```python
from build123d import *

# Parameters (mm, degrees)
EXTRUDE1_DEPTH             = 250
EXTRUDE2_REACH             = 252.125
SKETCH2_R                  = 1.75
SKETCH_R                   = 3
SKETCH_R_2                 = 1.75
EXTRUDE4_DEPTH             = 3.5
CHAMFER1_SIZE              = 0.2
LPATTERN1_COUNT            = 13
LPATTERN1_PITCH            = 20
CHAMFER1_OF_LPATTERN1_SIZE = 0.2


with BuildPart() as part:
    # Sketch1 → Extrude1 (new body)
    with BuildSketch(Plane.XY):
        with BuildLine():
            Line((-4.3, -3.25), (4.3, -3.25))
            Line((4.3, -3.25), (4.5, -3.05))
            Line((4.5, -3.05), (4.5, 0.455012563))
            ThreePointArc((4.5, 0.455012563), (3.924845827, 0.712323349), (3.617735397, 1.2625))
            Line((3.617735397, 1.2625), (3.15008224, 1.2625))
            Line((3.15008224, 1.2625), (3.15008224, 1.7625))
            Line((3.15008224, 1.7625), (3.65008224, 1.7625))
            ThreePointArc((3.65008224, 1.7625), (3.973877727, 2.229724887), (4.5, 2.444987437))
            Line((4.5, 2.444987437), (4.5, 3.05))
            Line((4.5, 3.05), (4.3, 3.25))
            Line((4.3, 3.25), (-4.3, 3.25))
            Line((-4.3, 3.25), (-4.5, 3.05))
            Line((-4.5, 3.05), (-4.5, 2.444987437))
            ThreePointArc((-4.5, 2.444987437), (-3.973877727, 2.229724887), (-3.65008224, 1.7625))
            Line((-3.65008224, 1.7625), (-3.15008224, 1.7625))
            Line((-3.15008224, 1.7625), (-3.15008224, 1.2625))
            Line((-3.15008224, 1.2625), (-3.617735397, 1.2625))
            ThreePointArc((-3.617735397, 1.2625), (-3.924845827, 0.712323349), (-4.5, 0.455012563))
            Line((-4.5, 0.455012563), (-4.5, -3.05))
            Line((-4.5, -3.05), (-4.3, -3.25))
        make_face()
    extrude(amount=EXTRUDE1_DEPTH)

    # Sketch2 → Extrude2 (cut, up to next)
    with BuildSketch(Plane(origin=(0, 3.25, 0), x_dir=(1, 0, 0), z_dir=(0, 1, 0)), mode=Mode.PRIVATE) as extrude2_sk1:
        with Locations(Location((0, -5, 0), (0, 0, 270))):
            Circle(SKETCH2_R)
    extrude2_tool1 = extrude(extrude2_sk1.sketch, amount=-EXTRUDE2_REACH, mode=Mode.PRIVATE) & part.part
    extrude2 = extrude2_tool1.solids().sort_by_distance((0, 3.25, 5))[0]
    add(extrude2, mode=Mode.SUBTRACT)

    # Sketch → Extrude4 (cut)
    with BuildSketch(Plane(origin=(0, 3.25, 0), x_dir=(1, 0, 0), z_dir=(0, 1, 0))):
        with Locations(Location((0, -5, 0), (0, 0, 270))):
            Circle(SKETCH_R)
        with Locations(Location((0, -5, 0), (0, 0, 270))):
            Circle(SKETCH_R_2, mode=Mode.SUBTRACT)
    extrude4 = extrude(amount=-EXTRUDE4_DEPTH, mode=Mode.SUBTRACT)

    # Chamfer1
    chamfer1_edges = [part.edges().sort_by_distance(p)[0] for p in [
        (0, -3.25, 3.25),
        (0, 3.25, 2),
    ]]
    chamfer(chamfer1_edges, length=CHAMFER1_SIZE)

    # LPattern1: Extrude2, Extrude4 ×13
    with Locations(*[(0, 0, i * LPATTERN1_PITCH) for i in range(1, LPATTERN1_COUNT)]):
        add(extrude2, mode=Mode.SUBTRACT)
        add(extrude4, mode=Mode.SUBTRACT)

    # Chamfer1 of LPattern1
    chamfer1_of_lpattern1_edges = [part.edges().sort_by_distance(p)[0] for p in [
        (0, -3.25, 23.25),
        (0, 3.25, 22),
        (0, -3.25, 43.25),
        (0, 3.25, 42),
        (0, -3.25, 63.25),
        (0, 3.25, 62),
        (0, -3.25, 83.25),
        (0, 3.25, 82),
        (0, -3.25, 103.25),
        (0, 3.25, 102),
        (0, -3.25, 123.25),
        (0, 3.25, 122),
        (0, -3.25, 143.25),
        (0, 3.25, 142),
        (0, -3.25, 163.25),
        (0, 3.25, 162),
        (0, -3.25, 183.25),
        (0, 3.25, 182),
        (0, -3.25, 203.25),
        (0, 3.25, 202),
        (0, -3.25, 223.25),
        (0, 3.25, 222),
        (0, -3.25, 243.25),
        (0, 3.25, 242),
    ]]
    chamfer(chamfer1_of_lpattern1_edges, length=CHAMFER1_OF_LPATTERN1_SIZE)


solid = part.part
```
Here's how the part is built. I have some questions about the finished solid (model axes, mm). Coordinates: 2 decimals unless noted, no trailing zeros. Answer as a JSON object with one key per item and string values. Group by question number.
(1) I need wall thicknesses on probe 1 along Y at (x, z) = (3.25, 54.5); probe 2 along X at (y, z) = (-1.7, 25); probe 3 along X at (y, z) = (1.35, 65). Which ranges of each line are inside material? Lowest first, please.
(2) Suppose I cut it at A-A, the plane x = 0. State how many separate pieces and enclosed holes the cut face has, then the cut area to 3 significant figures.
(3) For pin 1 (4 mm diameter, centred on x = 0, z = 105, fed in from +Y); pin 2 (3 mm diameter, centred on x = 0, z = 65, fed in from +Y), each with a flat end and sliding along its axis, tell me the tip position at first contact or that it passes through.
(4) If we mould it in two halves opening along Z, with no side actions, what happens to faces 1 (the face through (0, 1, 242)), 2 (the face through (0, 0, 0))? For each: released by +Z, released by -Z, zero draft, split by the parting line, or undercut.
Values found:
{
 "1": {"probe 1": "y = -3.25 to 1.26, 1.76 to 3.25", "probe 2": "x = -4.5 to -1.75, 1.75 to 4.5", "probe 3": "x = -3.15 to -3, 3 to 3.15"},
 "2": {"separate pieces": "14", "enclosed holes": "0", "area": "1,210 mm^2"},
 "3": {"pin 1": "stops at y = -0.25", "pin 2": "passes through"},
 "4": {"face 1": "undercut", "face 2": "released by -Z"}
}
